Can you work these out from the model? Positions are in its coordinate system, mm. Face numbers are marked on the shaded views. A direction names the side the tool comes from. Give positions to 0.01 mm unless a question says otherwise; leave off trailing zeros. Order: outer loops, then holes, each group sorted by start corner. A loop starts at its lowest first (then second) coordinate and runs counter-clockwise, first axis right, second up. Notation, with made-up numbers: (60.5, 39.25) -> (69.5, 39.25) arc R23 cw to (69.5, 55.25) -> close; hole circle Ø1 at (33.25, 36.5). An arc over 180 degrees is marked (long way). Answer as CSV lines item,"result".
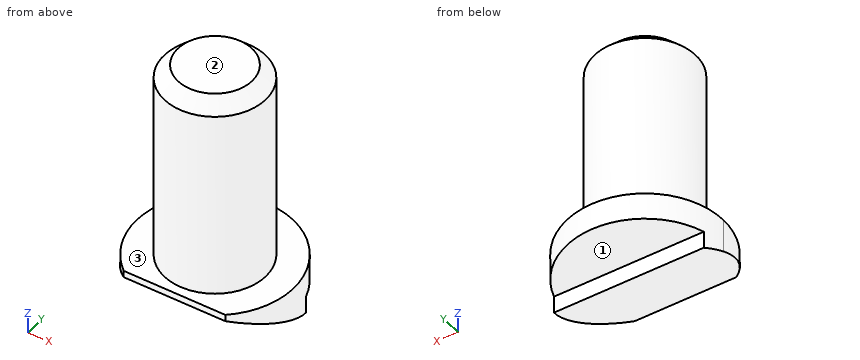
```python
from build123d import *

# Parameters (mm, degrees)
SKETCH_1_R          = 3.725
EXTRUDE_1_DEPTH     = 15
EXTRUDE_START       = 5
SKETCH_2_R          = 3.725
EXTRUDE_2_DEPTH     = 5
CHAMFER_2_SIZE      = 1
CHAMFER_3_SIZE      = 4.5
CHAMFER_3_SIZE2     = 10
CUT_EXTRUDE_1_DEPTH = 3


with BuildPart() as part:
    # 스케치1 → 보스-돌출1 (new body)
    with BuildSketch(Plane.XY):
        Circle(SKETCH_1_R)
    extrude(amount=EXTRUDE_1_DEPTH)

    # 스케치2 → 보스-돌출2 (add)
    # profile 1 of 2: a face of its own
    with BuildSketch(Plane(origin=(0, 0, 0), x_dir=(-1, 0, 0), z_dir=(0, 0, -1)).offset(EXTRUDE_START)):
        with BuildLine():
            ThreePointArc((5.75, 0), (-2.419672395, 5.216098686), (-3.713542783, -4.39))
            Line((-3.713542783, -4.39), (3.713542783, -4.39))
            ThreePointArc((3.713542783, -4.39), (5.216098686, -2.419672395), (5.75, 0))
        make_face()
        Circle(SKETCH_2_R, mode=Mode.SUBTRACT)
    # profile 2 of 2: a face of its own
    with BuildSketch(Plane(origin=(0, 0, 0), x_dir=(-1, 0, 0), z_dir=(0, 0, -1)).offset(EXTRUDE_START)):
        Circle(SKETCH_2_R)
    extrude(amount=-EXTRUDE_2_DEPTH)

    # 모따기2
    chamfer_2_edges = [part.edges().sort_by_distance(p)[0] for p in [
        (-3.725, 0, 15),
    ]]
    chamfer(chamfer_2_edges, length=CHAMFER_2_SIZE)

    # 모따기3
    chamfer_3_edges = [part.edges().sort_by_distance(p)[0] for p in [
        (0, -4.39, -5),
    ]]
    chamfer_3_side = [part.faces().sort_by_distance(p)[0] for p in [
        (0, -4.39, -2.5),
    ]]
    chamfer(chamfer_3_edges, length=CHAMFER_3_SIZE, length2=CHAMFER_3_SIZE2, reference=chamfer_3_side[0])

    # 스케치3 → 컷-돌출1 (cut)
    with BuildSketch(Plane(origin=(0, 0, -5), x_dir=(-1, 0, 0), z_dir=(0, 0, -1))):
        with BuildLine():
            ThreePointArc((-1.261110622, 5.61), (-3.882807448, 4.241026565), (-5.477225575, 1.75))
            Line((-5.477225575, 1.75), (5.477225575, 1.75))
            ThreePointArc((5.477225575, 1.75), (3.882807448, 4.241026565), (1.261110622, 5.61))
            Line((1.261110622, 5.61), (-1.261110622, 5.61))
        make_face()
        with BuildLine():
            Line((-1.261110622, 5.61), (1.261110622, 5.61))
            ThreePointArc((1.261110622, 5.61), (0, 5.75), (-1.261110622, 5.61))
        make_face()
    extrude(amount=-CUT_EXTRUDE_1_DEPTH, mode=Mode.SUBTRACT)


solid = part.part
```
Item 1: Imagine slicing it at D-D, the plane x = 4. Please give me the cut outline in (y, z), then the cut area to 3 significant figures.
Numbers:
outline,"(-4.13, -0.62) -> (1.75, -3.26) -> (1.75, -2) -> (4.13, -2) -> (4.13, 0) -> (-4.13, 0) -> close"
area,"16.2 mm²"
Item 2: For the marked faces 1, 2 and 3, which set-ups out of +Z, -Z, +X, -X, +Y, -Y let a thin tool reach every point of the face, with its end or its side?
Numbers:
face 1,"-Z, +X, -X, +Y"
face 2,"+Z, +X, -X, +Y, -Y"
face 3,"+Z"
Item 3: Imagine slicing it at A-A, the plane x = 0. Please give me the cut outline in (y, z) (3 decimals), then the cut area to 3 significant figures.
Numbers:
outline,"(-4.39, -0.5) -> (1.75, -3.263) -> (1.75, -2) -> (5.75, -2) -> (5.75, 0) -> (3.725, 0) -> (3.725, 14) -> (2.725, 15) -> (-2.725, 15) -> (-3.725, 14) -> (-3.725, 0) -> (-4.39, 0) -> close"
area,"130 mm²"
Item 4: Imagine slicing it at B-B, the plane z = 7.5. Please give me the cut outline in (x, y) (3 decimals), then the cut area to 3 significant figures.
Numbers:
outline,"circle Ø7.45 at (0, 0)"
area,"43.6 mm²"
Item 5: For pin 1 (0.6 mm diameter, centred on x = 2.5, z = -2.5, fed in from +Y); pin 2 (1 mm diameter, centred on x = -3.5, y = -2, fed in from +Z); pin 3 (6 mm diameter, centred on y = 3, z = 1, fed in from +X), each with a flat end and sliding along its axis, tell me the tip position at first contact or that it passes through.
Numbers:
pin 1,"stops at y = 1.75"
pin 2,"stops at z = 14.19"
pin 3,"stops at x = 5.75"
Item 6: Imagine slicing it at C-C, the plane y = 5. Please give me the cut outline in (x, z).
Numbers:
outline,"(-2.84, -2) -> (2.84, -2) -> (2.84, 0) -> (-2.84, 0) -> close"
Item 7: Please list where these lines run through material, in increasing order: line 1 along Z through (x, y) = (-1.25, 2); line 2 along Z through (x, y) = (0.75, 4); line 3 along Y through (x, z) = (-5, -2.25).
Numbers:
line 1,"z = -2 to 15"
line 2,"z = -2 to 0"
line 3,"y = -0.5 to 1.75"
